```python
from build123d import *

# Parameters (mm, degrees)
SKETCH1_W               = 10
SKETCH1_H               = 7.6
EXTRUDE1_DEPTH          = 10
SKETCH2_OUTSIDE_W       = 12.81
SKETCH2_OUTSIDE_H       = 15.21
CUT_EXTRUDE1_DEPTH      = 6
CUT_EXTRUDE1_DEPTH_BACK = 6
SKETCH3_R               = 1.65
SKETCH3_R_2             = 0.35
SKETCH3_W               = 0.4
SKETCH3_H               = 4
CUT_EXTRUDE2_DEPTH      = 4
SKETCH4_W               = 4
SKETCH4_H               = 5.5
CUT_EXTRUDE3_DEPTH      = 5.6
SKETCH5_W               = 4
SKETCH5_H               = 5.1
EXTRUDE2_DEPTH          = 4.25
SKETCH6_R               = 1.6
CUT_EXTRUDE4_DEPTH      = 4.25
EXTRUDE3_DEPTH          = 6.5
CUT_EXTRUDE5_DEPTH      = 6.5
SKETCH10_W              = 1.1
SKETCH10_H              = 0.5
CUT_EXTRUDE6_DEPTH      = 3.6
SKETCH11_R              = 0.5
EXTRUDE4_DEPTH          = 3.5
SKETCH12_R              = 1.65
EXTRUDE5_DEPTH          = 3
CUT_EXTRUDE7_DEPTH      = 0.4
EXTRUDE6_DEPTH          = 0.945
EXTRUDE9_DEPTH          = 0.39
LPATTERN1_COUNT         = 2
LPATTERN1_PITCH         = 5
FILLET1_R               = 0.3
FILLET2_R               = 0.7


with BuildPart() as part:
    # Sketch1 → Extrude1 (new body)
    with BuildSketch(Plane(origin=(0, 0, 0), x_dir=(1, 0, 0), z_dir=(0, 1, 0))):
        Rectangle(SKETCH1_W, SKETCH1_H)
    extrude(amount=EXTRUDE1_DEPTH)

    # Sketch2 outside → Cut-Extrude1 (cut, two sides)
    with BuildSketch(Plane(origin=(0, 0, 0), x_dir=(0, 0, -1), z_dir=(1, 0, 0))) as cut_extrude1_sk:
        with Locations((0, 5)):
            Rectangle(SKETCH2_OUTSIDE_W, SKETCH2_OUTSIDE_H)
        Polygon((2.5, 10), (3.8, 6.5), (3.8, 0), (-3.8, 0), (-3.8, 6.5), (-2.5, 10), align=None, mode=Mode.SUBTRACT)
    extrude(amount=CUT_EXTRUDE1_DEPTH, mode=Mode.SUBTRACT)
    extrude(cut_extrude1_sk.sketch, amount=-CUT_EXTRUDE1_DEPTH_BACK, mode=Mode.SUBTRACT)

    # Sketch3 → Cut-Extrude2 (cut)
    with BuildSketch(Plane(origin=(0, 10, 0), x_dir=(-1, 0, 0), z_dir=(0, 1, 0))):
        with Locations((2.5, 0)):
            Circle(SKETCH3_R)
        with Locations((-2.5, 0)):
            Circle(SKETCH3_R)
        with Locations((2.5, -2.78)):
            Circle(SKETCH3_R_2)
        with Locations((-2.5, -2.78)):
            Circle(SKETCH3_R_2)
        Rectangle(SKETCH3_W, SKETCH3_H)
    extrude(amount=-CUT_EXTRUDE2_DEPTH, mode=Mode.SUBTRACT)

    # Sketch4 → Cut-Extrude3 (cut)
    with BuildSketch(Plane.XY.offset(3.8)):
        with Locations((-2.5, 3.25)):
            Rectangle(SKETCH4_W, SKETCH4_H)
        with Locations((2.5, 3.25)):
            Rectangle(SKETCH4_W, SKETCH4_H)
    extrude(amount=-CUT_EXTRUDE3_DEPTH, mode=Mode.SUBTRACT)

    # Sketch5 → Extrude2 (add)
    with BuildSketch(Plane.XY.offset(-1.8)):
        with Locations((-2.5, 3.05)):
            Rectangle(SKETCH5_W, SKETCH5_H)
        with Locations((2.5, 3.05)):
            Rectangle(SKETCH5_W, SKETCH5_H)
    extrude(amount=EXTRUDE2_DEPTH)

    # Sketch6 → Cut-Extrude4 (cut)
    with BuildSketch(Plane.XY.offset(2.45)):
        with Locations((-2.5, 2.554263468)):
            Circle(SKETCH6_R)
        with Locations((2.5, 2.554263468)):
            Circle(SKETCH6_R)
    extrude(amount=-CUT_EXTRUDE4_DEPTH, mode=Mode.SUBTRACT)

    # Sketch7 → Extrude3 (add)
    with BuildSketch(Plane(origin=(0, 0, 0), x_dir=(1, 0, 0), z_dir=(0, 1, 0))):
        Polygon((-5.6, 3.1), (-5, 2.881617859), (-5, 2.118382141), (-5.6, 1.9), align=None)
    extrude(amount=EXTRUDE3_DEPTH)

    # Sketch9 → Cut-Extrude5 (cut)
    with BuildSketch(Plane(origin=(0, 0, 0), x_dir=(1, 0, 0), z_dir=(0, 1, 0))):
        Polygon((5, 2.881617859), (4.4, 3.1), (4.4, 1.9), (5, 2.118382141), align=None)
    extrude(amount=CUT_EXTRUDE5_DEPTH, mode=Mode.SUBTRACT)

    # Sketch10 → Cut-Extrude6 (cut)
    with BuildSketch(Plane.XY.offset(3.8)):
        with Locations((-2.5, 0.25)):
            Rectangle(SKETCH10_W, SKETCH10_H)
        with Locations((2.5, 0.25)):
            Rectangle(SKETCH10_W, SKETCH10_H)
    extrude(amount=-CUT_EXTRUDE6_DEPTH, mode=Mode.SUBTRACT)

    # Sketch11 → Extrude4 (add)
    with BuildSketch(Plane.XZ.offset(-0.5)):
        with Locations((-2.5, 0.8)):
            Circle(SKETCH11_R)
        with Locations((2.5, 0.8)):
            Circle(SKETCH11_R)
    extrude(amount=EXTRUDE4_DEPTH)

    # Sketch12 → Extrude5 (add)
    with BuildSketch(Plane.XZ.offset(-6)):
        with Locations((2.5, 0)):
            Circle(SKETCH12_R)
        with Locations((-2.5, 0)):
            Circle(SKETCH12_R)
    extrude(amount=-EXTRUDE5_DEPTH)

    # Sketch13 → Cut-Extrude7 (cut)
    with BuildSketch(Plane(origin=(0, 9, 0), x_dir=(-1, 0, 0), z_dir=(0, 1, 0))):
        with BuildLine():
            Line((3.594307251, -1.234905519), (1.825829895, 1.505986278))
            ThreePointArc((1.825829895, 1.505986278), (1.605433494, 1.386452583), (1.405692749, 1.234905519))
            Line((1.405692749, 1.234905519), (3.174170105, -1.505986278))
            ThreePointArc((3.174170105, -1.505986278), (3.394566506, -1.386452583), (3.594307251, -1.234905519))
        make_face()
        with BuildLine():
            Line((-2.83217089, -1.616218581), (-1.698971441, 1.44251629))
            ThreePointArc((-1.698971441, 1.44251629), (-1.926782442, 1.54723031), (-2.16782911, 1.616218581))
            Line((-2.16782911, 1.616218581), (-3.301028559, -1.44251629))
            ThreePointArc((-3.301028559, -1.44251629), (-3.073217558, -1.54723031), (-2.83217089, -1.616218581))
        make_face()
    extrude(amount=-CUT_EXTRUDE7_DEPTH, mode=Mode.SUBTRACT)

    # Sketch14 → Extrude6 (add, symmetric)
    with BuildSketch(Plane.ZY.offset(2.5)):
        Polygon((2.45, 5.6), (3.03887637, 3.861674443), (0.167170254, 1.787608865), (-0.546359637, 2.097431054), (-0.705673534, 1.730526322), (0.216750724, 1.33), (3.512480259, 3.710312924), (2.736824279, 6), (-1.8, 6), (-1.8, 5.6), align=None)
    extrude6 = extrude(amount=EXTRUDE6_DEPTH, both=True)

    # Sketch15 → Extrude9 (add)
    with BuildSketch(Plane(origin=(0, 1.449355072, 4.278403908), x_dir=(1, 0, 0), z_dir=(0, 0.320850379, 0.947129893))):
        Polygon((-1.555, 4.8), (-1.555, 2.903968921), (-0.51, 4.8), align=None)
        Polygon((-3.445, 4.8), (-3.445, 2.903968921), (-4.49, 4.8), align=None)
    extrude9 = extrude(amount=-EXTRUDE9_DEPTH)

    # LPattern1: Extrude6, Extrude9 ×2
    with Locations(*[(i * LPATTERN1_PITCH, 0, 0) for i in range(1, LPATTERN1_COUNT)]):
        add(extrude6)
        add(extrude9)

    # Fillet1
    fillet1_edges = [part.edges().sort_by_distance(p)[0] for p in [
        (-2.5, 3.861674443, 3.03887637),
        (-2.5, 1.787608865, 0.167170254),
        (2.5, 3.861674443, 3.03887637),
        (2.5, 1.787608865, 0.167170254),
    ]]
    fillet(fillet1_edges, radius=FILLET1_R)

    # Fillet2
    fillet2_edges = [part.edges().sort_by_distance(p)[0] for p in [
        (-2.5, 3.710312924, 3.512480259),
        (-2.5, 1.33, 0.216750724),
        (2.5, 1.33, 0.216750724),
        (2.5, 3.710312924, 3.512480259),
    ]]
    fillet(fillet2_edges, radius=FILLET2_R)


solid = part.part
```
Geometry check sheet. Reference: the model listing, model coordinates, mm. A direction names the side the tool comes from. Round coordinates to 2 decimals unless told otherwise and drop trailing zeros. Order: outer loops, then holes, each group sorted by start corner. A loop starts at its lowest first (then second) coordinate and runs counter-clockwise, first axis right, second up. Notation, with made-up numbers: (-38.75, -7) -> (-19.75, -7) arc R23 ccw to (-19.75, 9) -> close; hole circle Ø2 at (20.25, 71). An arc over 180 degrees is marked (long way). Return JSON: item names as keys, results as strings. Group by question number.
Q1. Tool access check on faces 1 (the flat face through (2.726, 8.803, 0.108)), 2 (the flat face through (4, 5.6, 0)), 3 (the flat face through (-1, 0.5, 3)), 4 (the cylindrical face through (2.392, -1.226, 0.312)). Record the directions out of +Z, -Z, +X, -X, +Y, -Y that give a thin tool (end or side, any length) a straight path to the whole face; none if there is none.
Q2. Release check for a two-part mould opening along Z. For faces 5 (the flat face through (3.96, 5.02, 2.86)), 6 (the flat face through (3, 9, 0)), 7 (the flat face through (5, 5, 0)) record: released by +Z, released by -Z, zero draft, split by the parting line, or undercut.
Q3. Gauge pin test, flat ends, axial feed: pin 1 (2.5 mm diameter, centred on x = -2, y = 2, fed in from +Z); pin 2 (4 mm diameter, centred on x = -1.5, y = -1, fed in from +Z); pin 3 (3 mm diameter, centred on x = 4, y = 8.5, fed in from -Z); pin 4 (1.2 mm diameter, centred on x = -2.5, z = -0.5, fed in from +Y). Record the tip position at first contact, or that the pin passes through.
Q4. Section check A-A, the plane x = 3.75. Record the boundary of the cut face in (y, z).
Q5. Material ranges on probe 1 along X at (y, z) = (9.7, 0); probe 2 along Y at (x, z) = (-3.75, 2.25); probe 3 along Y at (x, z) = (-3.5, -1.5), recorded low to high. Write a range as from..to.
Q6. Section check C-C, the plane y = 7.5. Record the boundary of the cut face in (x, z).
Q7. Section check B-B, the plane z = 0.8. Count the separate pieces of the cut face and the enclosed holes in it, plus the area to 3 significant figures.
Numbers:
{
 "1": {"face 1": "+Y", "face 2": "none", "face 3": "+Z", "face 4": "-Y"},
 "2": {"face 5": "released by +Z", "face 6": "undercut", "face 7": "zero draft"},
 "3": {"pin 1": "z = 2.88", "pin 2": "z = 3.8", "pin 3": "z = -3.61", "pin 4": "y = 9"},
 "4": {"outline": "(0, -3.8) -> (6.5, -3.8) -> (10, -2.5) -> (10, -1.08) -> (9, -1.08) -> (9, 1.08) -> (10, 1.08) -> (10, 2.5) -> (6.5, 3.8) -> (6, 3.8) -> (6, -1.8) -> (5.6, -1.8) -> (5.6, 2.45) -> (3.55, 2.45) -> (3.55, -1.8) -> (1.56, -1.8) -> (1.56, 2.45) -> (0.5, 2.45) -> (0.5, 3.8) -> (0, 3.8) -> close; (4.6, 2.8) -> (5.87, 2.37) -> (6, 2.74) -> (4.72, 3.17) -> close"},
 "5": {"probe 1": "-5..-4.15, -0.85..-0.2, 0.2..0.85, 4.15..5", "probe 2": "0..1.56, 3.55..5.6, 6..10", "probe 3": "0..1.31, 3.8..5.6, 6..10"},
 "6": {"outline": "(-5, -3.43) -> (5, -3.43) -> (5, 3.43) -> (-5, 3.43) -> close; hole circle Ø0.7 at (-2.5, -2.78); hole (-0.2, -2) -> (0.2, -2) -> (0.2, 2) -> (-0.2, 2) -> close; hole circle Ø0.7 at (2.5, -2.78)"},
 "7": {"separate pieces": "3", "enclosed holes": "6", "area": "82.2 mm^2"}
}
